Geometry: final body of the model. Coordinates: model frame, mm. A direction names the side the tool comes from. Give positions to 0.01 mm unless a question says otherwise; leave off trailing zeros. Use a Markdown table: item, result. Add a question column.
1) Pin query (flat end, axial travel): pin 1 (3 mm diameter, centred on x = -29.5, z = 1, fed in from -Y). Return the tip coordinate at first contact, or that it passes through.
2) Set-up query: faces 1 (the flat face through (65.088, 13, 2)), 2 (the flat face through (63, 13, 25.4)), 3 (the flat face through (-63, 13, 29.464)). Return all of +Z, -Z, +X, -X, +Y, -Y with unobstructed straight access to the full face (end or side cutting, diameter ignored); none if empty.
3) Line query: line 1 (X direction, y = 23.25, z = -23.5); line 2 (X direction, y = 22, z = -23). Output: solid intervals per line, ascending.
```python
from build123d import *

# Parameters (mm, degrees)
SKETCH1_W           = 130.175
SKETCH1_H           = 76.2
BOSS_EXTRUDE1_DEPTH = 25.4
CUT_EXTRUDE1_DEPTH  = 26.4


with BuildPart() as part:
    # Sketch1 → Boss-Extrude1 (new body)
    with BuildSketch(Plane(origin=(0, 0, 0), x_dir=(1, 0, 0), z_dir=(0, 1, 0))):
        Rectangle(SKETCH1_W, SKETCH1_H)
    extrude(amount=BOSS_EXTRUDE1_DEPTH)

    # Sketch2 → Cut-Extrude1 (cut, through all)
    with BuildSketch(Plane(origin=(0, 25.4, 0), x_dir=(1, 0, 0), z_dir=(0, 1, 0))):
        with BuildLine():
            Line((-60.7695, 25.4), (-65.0875, 25.4))
            Line((-65.0875, 25.4), (-65.0875, 21.336))
            Line((-65.0875, 21.336), (-60.7695, 21.336))
            ThreePointArc((-60.7695, 21.336), (-58.7375, 23.368), (-60.7695, 25.4))
        make_face()
        with BuildLine():
            Line((-60.7695, -25.4), (-65.0875, -25.4))
            Line((-65.0875, -25.4), (-65.0875, -29.464))
            Line((-65.0875, -29.464), (-60.7695, -29.464))
            ThreePointArc((-60.7695, -29.464), (-58.7375, -27.432), (-60.7695, -25.4))
        make_face()
    cut_extrude1 = extrude(amount=-CUT_EXTRUDE1_DEPTH, mode=Mode.SUBTRACT)

    # Mirror2: Cut-Extrude1 across plane
    add(cut_extrude1.mirror(Plane(origin=(0, 0, 0), x_dir=(0, 0, 1), z_dir=(1, 0, 0))), mode=Mode.SUBTRACT)


solid = part.part
```
Found:
| question | item | result |
|---|---|---|
| 1 | pin 1 | y = 0 |
| 2 | face 1 | +Z, -Z, +X, +Y, -Y |
| 2 | face 2 | +X, +Y, -Y |
| 2 | face 3 | -X, +Y, -Y |
| 3 | line 1 | -58.74 to 58.74 |
| 3 | line 2 | -58.77 to 58.77 |
